For this review, use the dimensioned drawing (mm, ordinates from the lowest corner) and the shaded views. A direction names the side the tool comes from. Give positions to 0.01 mm unless a question says otherwise; leave off trailing zeros. Loops run counter-clockwise (first coordinate to the right, second up) from the corner with the lowest first, then second, coordinate; pieces in that order, holes last. Notation, with made-up numbers: M -6.5,-31 L -1.5,-31 A19 ccw -1.5,-5 Z; hole C 1.5,4 d4. An arc over 180 degrees is marked long. Use a Markdown table: item, result. Add a question column.
(1) Add section B-B, the plane z = 2.35. Give the boundary of the cut face in (x, y), then the cut area to 3 significant figures.
(2) Add section D-D, the plane x = 9. Give the boundary of the cut face in (y, z), then the cut area to 3 significant figures.
(3) For probe 1 along X at (y, z) = (2, 3.15); probe 2 along Y at (x, z) = (37.5, 2.55); probe 3 along Y at (x, z) = (8.5, 3.15), list the stretches that pass through material, from the lowest coordinate up.
(4) Add section C-C, the plane x = 2.5. Give the boundary of the cut face in (y, z), then the cut area to 3 significant figures.
(5) For the marked faces 4 and 5, list the 3-axis set-ups (+Z, -Z, +X, -X, +Y, -Y) from which the entire face can be reached by the end or side of a thin tool; tool diameter is ignored.
(6) Insertion check: pin 1 Ø6 at (x, y) = (17, 10.5) entering from +Z; pin 2 Ø1.4 at (x, y) = (37.5, 28) entering from -Z. Each pin has a flat end and moves straight along its axis. Give the tip position at first contact, or say it passes through.
(7) Draft analysis for pull direction Y (two halves, no side actions). For the marked faces 1, 2 and 3, state which applies: pulls with the +Y half, pulls with the -Y half, needs draft (parallel to the pull), parting line crosses it, or undercut.
(8) Add section A-A, the plane y = 2. Give the boundary of the cut face in (x, z).
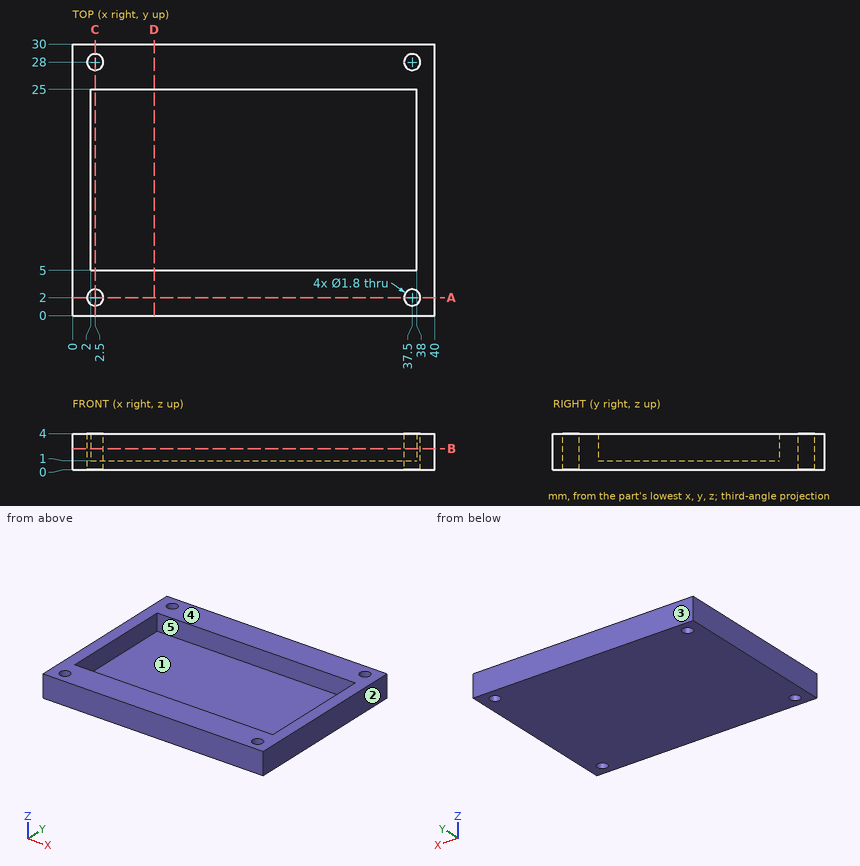
Established:
| question | item | result |
|---|---|---|
| 1 | outline | M 0,0 L 40,0 L 40,30 L 0,30 Z; hole C 2.5,2 d1.8; hole C 2.5,28 d1.8; hole M 2,5 L 38,5 L 38,25 L 2,25 Z; hole C 37.5,2 d1.8; hole C 37.5,28 d1.8 |
| 1 | area | 470 mm^2 |
| 2 | outline | M 0,0 L 30,0 L 30,4 L 25,4 L 25,1 L 5,1 L 5,4 L 0,4 Z |
| 2 | area | 60.0 mm^2 |
| 3 | probe 1 | 0 to 1.6, 3.4 to 36.6, 38.4 to 40 |
| 3 | probe 2 | 0 to 1.1, 2.9 to 5, 25 to 27.1, 28.9 to 30 |
| 3 | probe 3 | 0 to 5, 25 to 30 |
| 4 | outline | M 0,0 L 1.1,0 L 1.1,4 L 0,4 Z; M 2.9,0 L 27.1,0 L 27.1,4 L 25,4 L 25,1 L 5,1 L 5,4 L 2.9,4 Z; M 28.9,0 L 30,0 L 30,4 L 28.9,4 Z |
| 4 | area | 45.6 mm^2 |
| 5 | face 4 | +Z, +X, -X, +Y, -Y |
| 5 | face 5 | +Z |
| 6 | pin 1 | z = 1 |
| 6 | pin 2 | through |
| 7 | face 1 | undercut |
| 7 | face 2 | needs draft |
| 7 | face 3 | pulls with the +Y half |
| 8 | outline | M 0,0 L 1.6,0 L 1.6,4 L 0,4 Z; M 3.4,0 L 36.6,0 L 36.6,4 L 3.4,4 Z; M 38.4,0 L 40,0 L 40,4 L 38.4,4 Z |
